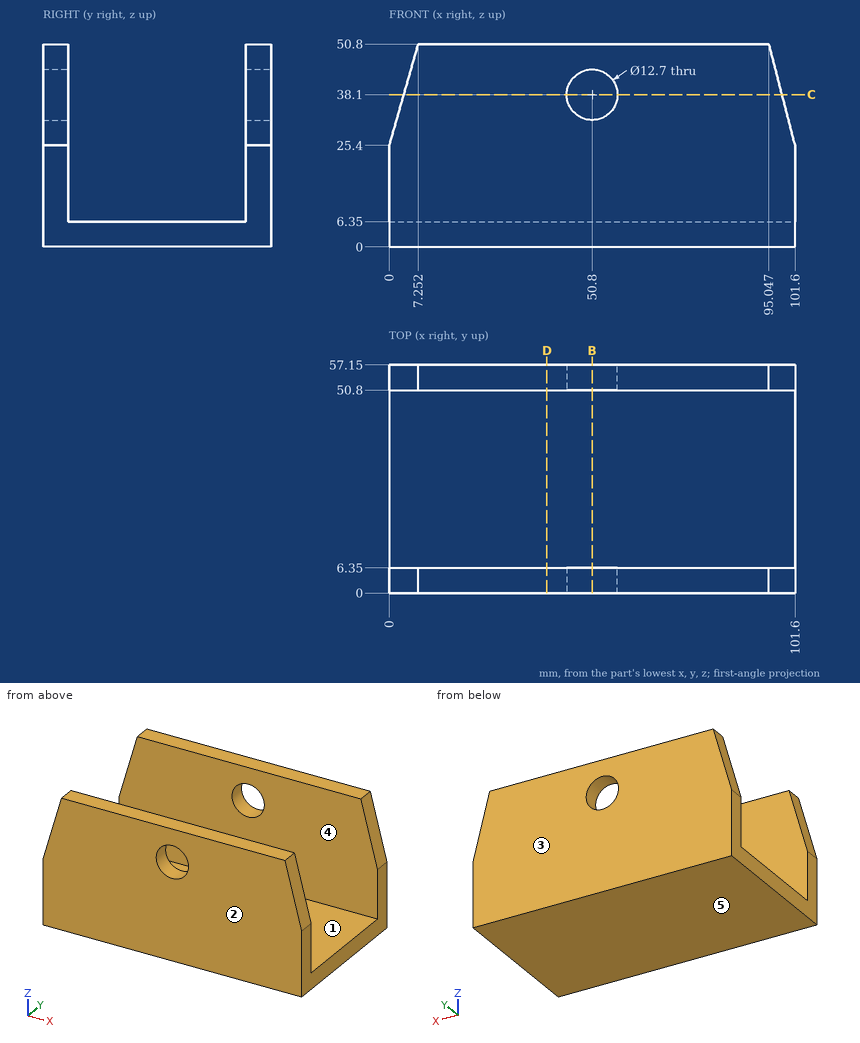
Geometry: see drawing. Coordinates: mm, zero at the bounding-box minimum. A direction names the side the tool comes from. Give positions to 0.01 mm unless a question says otherwise; leave off trailing zeros. Loops run counter-clockwise (first coordinate to the right, second up) from the corner with the lowest first, then second, coordinate; pieces in that order, holes last. Notation, with made-up numbers: M -25.5,19.25 L 26.5,19.25 A29 cw 26.5,41.25 Z; hole C -35,72 d8. An arc over 180 degrees is marked long. Use one line per item in the form item = value.
1. First-contact query: pin 1 (4 mm diameter, centred on x = 29, y = 15.5, fed in from +Z); pin 2 (7.5 mm diameter, centred on x = 50.8, z = 38.1, fed in from +Y). Flat tips, straight axial feed; report the tip coordinate or a pass-through.
Numbers:
pin_1 = 6.35
pin_2 = through
2. Section query C-C, the plane z = 38.1. Return the cut outline in (x, y).
Numbers:
outline = M 3.63,0 L 44.45,0 L 44.45,6.35 L 3.63,6.35 Z; M 3.63,50.8 L 44.45,50.8 L 44.45,57.15 L 3.63,57.15 Z; M 57.15,0 L 98.32,0 L 98.32,6.35 L 57.15,6.35 Z; M 57.15,50.8 L 98.32,50.8 L 98.32,57.15 L 57.15,57.15 Z
3. Line query: L1, parallel to Y at x = 83, z = 18.5; L2, parallel to Z at x = 50.8, y = 53.5. Output: solid intervals per line, ascending.
Numbers:
L1 = 0 to 6.35, 50.8 to 57.15
L2 = 0 to 31.75, 44.45 to 50.8
4. Section query D-D, the plane x = 39.5. Return the cut outline in (y, z).
Numbers:
outline = M 0,0 L 57.15,0 L 57.15,50.8 L 50.8,50.8 L 50.8,6.35 L 6.35,6.35 L 6.35,50.8 L 0,50.8 Z
5. Reachability of the marked faces 1 and 2 from +Z, -Z, +X, -X, +Y, -Y: full face, straight path, thin tool, end or side. Return the list, or none.
Numbers:
face_1 = +Z, +X, -X
face_2 = +Z, -Z, +X, -X, -Y
6. Pull-direction query (Y, two-part tool) for the marked faces 3, 4 and 5; classes: released by +Y, released by -Y, zero draft, split by the parting line, or undercut.
Numbers:
face_3 = released by +Y
face_4 = undercut
face_5 = zero draft
7. Section query B-B, the plane x = 50.8. Return the cut outline in (y, z), and give its area (3 significant figures).
Numbers:
outline = M 0,0 L 57.15,0 L 57.15,31.75 L 50.8,31.75 L 50.8,6.35 L 6.35,6.35 L 6.35,31.75 L 0,31.75 Z; M 0,44.45 L 6.35,44.45 L 6.35,50.8 L 0,50.8 Z; M 50.8,44.45 L 57.15,44.45 L 57.15,50.8 L 50.8,50.8 Z
area = 766 mm²
